```python
from build123d import *

# Parameters (mm, degrees)
BOSS_EXTRUDE1_DEPTH = 2.38125
SKETCH2_R           = 1.651
BOSS_EXTRUDE2_DEPTH = 0.79375


with BuildPart() as part:
    # Sketch1 → Boss-Extrude1 (new body)
    with BuildSketch(Plane(origin=(0, 0, 0), x_dir=(1, 0, 0), z_dir=(0, 1, 0))):
        with BuildLine():
            Line((-6.355837102, -10.127283918), (6.344162898, -10.127283918))
            Line((6.344162898, -10.127283918), (6.344162898, -45.052283918))
            ThreePointArc((6.344162898, -45.052283918), (-0.005837102, -45.693764185), (-6.355837102, -45.052283918))
            Line((-6.355837102, -45.052283918), (-6.355837102, -10.127283918))
        make_face()
        Polygon((3.181862898, -25.055183638), (3.181862898, -21.374344732), (-0.005837102, -19.533925278), (-3.193537102, -21.374344732), (-3.193537102, -25.055183638), (-0.005837102, -26.895603091), align=None, mode=Mode.SUBTRACT)
        Polygon((3.181862898, -37.374183638), (3.181862898, -33.693344732), (-0.005837102, -31.852925278), (-3.193537102, -33.693344732), (-3.193537102, -37.374183638), (-0.005837102, -39.214603091), align=None, mode=Mode.SUBTRACT)
    extrude(amount=BOSS_EXTRUDE1_DEPTH)

    # Sketch2 → Boss-Extrude2 (add)
    with BuildSketch(Plane(origin=(0, 2.38125, 0), x_dir=(1, 0, 0), z_dir=(0, 1, 0))):
        with BuildLine():
            Line((6.344162898, -45.052283918), (6.344162898, -10.127283918))
            Line((6.344162898, -10.127283918), (-6.355837102, -10.127283918))
            Line((-6.355837102, -10.127283918), (-6.355837102, -45.052283918))
            ThreePointArc((-6.355837102, -45.052283918), (-0.005837102, -45.693764185), (6.344162898, -45.052283918))
        make_face()
        with Locations((-0.005837102, -23.214764185)):
            Circle(SKETCH2_R, mode=Mode.SUBTRACT)
        with Locations((-0.005837102, -35.533764185)):
            Circle(SKETCH2_R, mode=Mode.SUBTRACT)
    extrude(amount=BOSS_EXTRUDE2_DEPTH)


solid = part.part
```
Can you work these out from the model? Positions are in its coordinate system, mm. A direction names the side the tool comes from. Round coordinates to 2 decimals unless told otherwise and drop trailing zeros. Loops run counter-clockwise (first coordinate to the right, second up) from the corner with the lowest first, then second, coordinate; pieces in that order, holes last. Notation, with made-up numbers: M 74.5,-6.5 L 133.5,-6.5 A6 ccw 133.5,-1.5 Z; hole C -7,-15 d1. An arc over 180 degrees is marked long. Answer as a JSON object with one key per item and string values. Group by question number.
Q1. We'd pull the mould along Z, two halves only. Please class faces 1 (the flat face through (1.61, 1.174, 20.467)), 2 (the flat face through (0, 2, 10.127)), 3 (the flat face through (0, 0, 28)): +Z half, -Z half, draft (parallel to the pull), parting line (faces both ways), or undercut.
Q2. Imagine slicing it at A-A, the plane y = 1.7. Please give me the cut outline in (x, z), then the cut area to 3 significant figures.
Q3. Imagine slicing it at C-C, the plane z = 24. Please give me the cut outline in (x, y) (3 decimals), then the cut area to 3 significant figures.
Q4. On a 3-axis mill with a long thin cutter (end or side, diameter ignored), from which of +Z, -Z, +X, -X, +Y, -Y can I reach the whole of each face in a straight line? I mean faces 4 (the cylindrical face through (-0.095, 1.565, 45.694)), 5 (the flat face through (-3.194, 1, 23)). Say none if no direction works.
Q5. Please list where these lines run through material, in increasing order: L1, parallel to Z at x = 0, y = 1.1; L2, parallel to X at y = 0.65, z = 24.5; L3, parallel to Z at x = -3, y = 1.9.
Q6. Imagine slicing it at D-D, the plane x = -2. Please give me the cut outline in (y, z) (3 decimals).
Q7. Imagine slicing it at B-B, the plane x = 0.5. Please give me the cut outline in (y, z) (3 decimals).
Q8. Will this pin go through, and if not, where does the flat tip stop? pin 1 (3 mm diameter, centred on x = -0.5, z = 37, fed in from -Y).
Findings:
{
 "1": {"face 1": "undercut", "face 2": "-Z half", "face 3": "draft"},
 "2": {"outline": "M -6.36,10.13 L 6.34,10.13 L 6.34,45.05 A31.75 ccw -6.36,45.05 Z; hole M -3.19,21.37 L -0.01,19.53 L 3.18,21.37 L 3.18,25.06 L -0.01,26.9 L -3.19,25.06 Z; hole M -3.19,33.69 L -0.01,31.85 L 3.18,33.69 L 3.18,37.37 L -0.01,39.21 L -3.19,37.37 Z", "area": "379 mm2"},
 "3": {"outline": "M -6.356,0 L -3.194,0 L -3.194,2.381 L -1.458,2.381 L -1.458,3.175 L -6.356,3.175 Z; M 1.446,2.381 L 3.182,2.381 L 3.182,0 L 6.344,0 L 6.344,3.175 L 1.446,3.175 Z", "area": "22.8 mm2"},
 "4": {"face 4": "+Z, +Y, -Y", "face 5": "-Y"},
 "5": {"L1": "z = 10.13 to 19.54, 26.89 to 31.86, 39.21 to 45.69", "L2": "x = -6.36 to -3.19, 3.18 to 6.34", "L3": "z = 10.13 to 21.26, 25.17 to 33.58, 37.49 to 45.55"},
 "6": {"outline": "M 0,10.127 L 3.175,10.127 L 3.175,45.631 L 0,45.631 L 0,38.063 L 2.381,38.063 L 2.381,33.004 L 0,33.004 L 0,25.744 L 2.381,25.744 L 2.381,20.685 L 0,20.685 Z"},
 "7": {"outline": "M 0,10.127 L 3.175,10.127 L 3.175,21.643 L 2.381,21.643 L 2.381,19.826 L 0,19.826 Z; M 0,26.604 L 2.381,26.604 L 2.381,24.786 L 3.175,24.786 L 3.175,33.962 L 2.381,33.962 L 2.381,32.145 L 0,32.145 Z; M 0,38.923 L 2.381,38.923 L 2.381,37.105 L 3.175,37.105 L 3.175,45.69 L 0,45.69 Z"},
 "8": {"pin 1": "stops at y = 2.38"}
}
